from build123d import *

# Parameters (mm, degrees)
BOX010_W     = 94
BOX010_H     = 94
BOX010_DEPTH = 2
FILLET011_R  = 7
BOX009_W     = 100
BOX009_H     = 100
BOX009_DEPTH = 2
FILLET010_R  = 7


with BuildPart() as top_with_fillets004:
    # Box010 → Box010 (new body)
    with BuildSketch(Plane(origin=(3, 3, 0), x_dir=(1, 0, 0), z_dir=(0, 0, 1))):
        with Locations((47, 47)):
            Rectangle(BOX010_W, BOX010_H)
    extrude(amount=BOX010_DEPTH)

    # Fillet011
    fillet011_edges = [top_with_fillets004.edges().sort_by_distance(p)[0] for p in [
        (3, 3, 1),
        (3, 97, 1),
        (97, 3, 1),
        (97, 97, 1),
    ]]
    fillet(fillet011_edges, radius=FILLET011_R)


with BuildPart() as stacker:
    # Box009 → Box009 (new body)
    with BuildSketch(Plane.XY):
        with Locations((50, 50)):
            Rectangle(BOX009_W, BOX009_H)
    extrude(amount=BOX009_DEPTH)

    # Fillet010
    fillet010_edges = [stacker.edges().sort_by_distance(p)[0] for p in [
        (0, 0, 1),
        (0, 100, 1),
        (100, 0, 1),
        (100, 100, 1),
    ]]
    fillet(fillet010_edges, radius=FILLET010_R)

    # Cut003: cut Top with fillets004
    add(top_with_fillets004.part, mode=Mode.SUBTRACT)


with BuildPart() as stacker_1:
    # Cut003 placement: moved
    add(stacker.part.moved(Location((0, 110, 0))))


solid = stacker_1.part
Input: part model. Units: mm. Frame: model coordinates. A direction names the side the tool comes from. Round coordinates to 2 decimals unless told otherwise and drop trailing zeros. Loops run counter-clockwise (first coordinate to the right, second up) from the corner with the lowest first, then second, coordinate; pieces in that order, holes last. Notation, with made-up numbers: (64, -30) -> (80, -30) arc R20 ccw to (80, 2) -> close; hole circle Ø8 at (20.25, 11). An arc over 180 degrees is marked (long way). Answer as a JSON object with one key per item and string values. Group by question number.
1) Ray query, L1, parallel to Y at x = 66.5, z = 1.8; L2, parallel to X at y = 131, z = 1.15; L3, parallel to X at y = 119, z = 0.3. Return the intervals inside material, ascending.
2) Draft query along Y for faces 1 (the flat face through (50, 112, 0)), 2 (the cylindrical face through (94.9, 115, 1)), 3 (the cylindrical face through (95, 204.9, 1)), 4 (the cylindrical face through (2, 112.1, 1)). Return one class per face: +Y half, -Y half, draft (parallel to the pull), parting line (faces both ways), or undercut.
3) Section query A-A on x = 68. Output: boundary loops of the cut face in (y, z), plus the area to 3 significant figures.
4) Reachability of faces 5 (the cylindrical face through (5, 115.1, 1)), 6 (the flat face through (50, 112, 2)) from +Z, -Z, +X, -X, +Y, -Y: full face, straight path, thin tool, end or side. Return the list, or none.
5) Section query B-B on y = 184.5. Output: boundary loops of the cut face in (x, z).
6) Section query C-C on z = 0.6. Output: boundary loops of the cut face in (x, y).
Reply:
{
 "1": {"L1": "y = 110 to 113, 207 to 210", "L2": "x = 0 to 3, 97 to 100", "L3": "x = 0 to 3.07, 96.93 to 100"},
 "2": {"face 1": "draft", "face 2": "undercut", "face 3": "undercut", "face 4": "-Y half"},
 "3": {"outline": "(110, 0) -> (113, 0) -> (113, 2) -> (110, 2) -> close; (207, 0) -> (210, 0) -> (210, 2) -> (207, 2) -> close", "area": "12.0 mm2"},
 "4": {"face 5": "+Z, -Z", "face 6": "+Z, +X, -X, +Y, -Y"},
 "5": {"outline": "(0, 0) -> (3, 0) -> (3, 2) -> (0, 2) -> close; (97, 0) -> (100, 0) -> (100, 2) -> (97, 2) -> close"},
 "6": {"outline": "(0, 117) arc R7 ccw to (7, 110) -> (93, 110) arc R7 ccw to (100, 117) -> (100, 203) arc R7 ccw to (93, 210) -> (7, 210) arc R7 ccw to (0, 203) -> close; hole (3, 120) arc R7 ccw to (10, 113) -> (90, 113) arc R7 ccw to (97, 120) -> (97, 200) arc R7 ccw to (90, 207) -> (10, 207) arc R7 ccw to (3, 200) -> close"}
}
